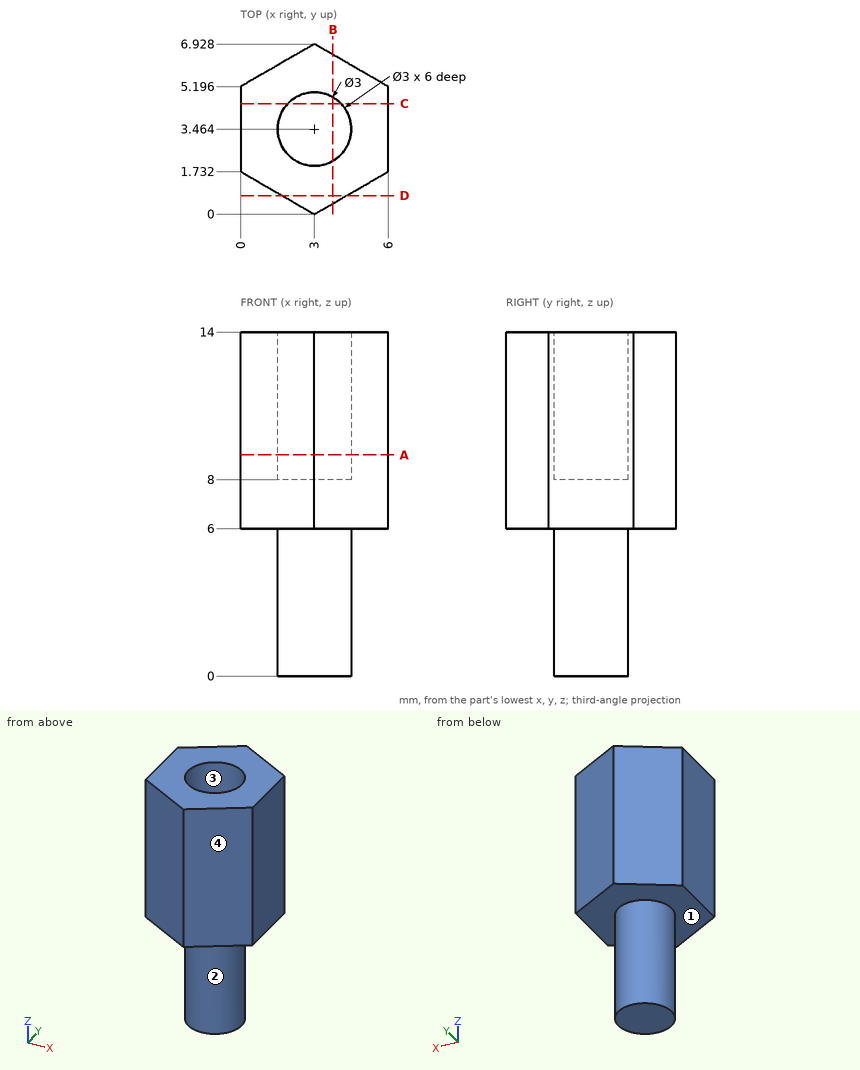
Geometry check sheet. Reference: drawing and pictorial views, mm from the part's lowest x, y, z. Coordinates: 2 decimals unless noted, no trailing zeros. Order: outer loops, then holes, each group sorted by start corner. A loop starts at its lowest first (then second) coordinate and runs counter-clockwise, first axis right, second up.
Item 1: Depth check by flat-ended pin: pin 1 (1.5 mm diameter, centred on x = 2.5, y = 3.5, fed in from +Z); pin 2 (1 mm diameter, centred on x = 1.5, y = 5.5, fed in from -Z). Enter the tip coordinate at first touch or a pass-through.
Item 2: Section check A-A (z = 9). Enter the section's corners in (x, y), plus the area to 3 significant figures.
Item 3: Mould release check, pull along X, two halves, no side actions. Record for the marked faces 1, 2, 3 and 4: released by +X, released by -X, zero draft, split by the parting line, or undercut.
Item 4: Section check B-B (x = 3.75). Enter the section's corners in (y, z) (1 decimal), plus the area to 3 significant figures.
Item 5: Section check D-D (y = 0.75). Enter the section's corners in (x, z).
Item 6: Section check C-C (y = 4.5). Enter the section's corners in (x, z) (1 decimal), plus the area to 3 significant figures.
Item 7: Scan lines: line 1 along Z through (x, y) = (0.5, 5); line 2 along X through (y, z) = (4.5, 8.5) (1 decimal); line 3 along Y through (x, z) = (3, 3.5). Record each from-to range of solid material in increasing order.
Check sheet entries:
1. pin 1: stops at z = 8
1. pin 2: stops at z = 6
2. outline: (0, 1.73) - (3, 0) - (6, 1.73) - (6, 5.2) - (3, 6.93) - (0, 5.2) - close; hole circle Ø3 at (3, 3.46)
2. area: 24.1 mm2
3. face 1: zero draft
3. face 2: split by the parting line
3. face 3: undercut
3. face 4: released by +X
4. outline: (0.4, 6) - (2.2, 6) - (2.2, 0) - (4.8, 0) - (4.8, 6) - (6.5, 6) - (6.5, 14) - (4.8, 14) - (4.8, 8) - (2.2, 8) - (2.2, 14) - (0.4, 14) - close
4. area: 48.5 mm2
5. outline: (1.7, 6) - (4.3, 6) - (4.3, 14) - (1.7, 14) - close
6. outline: (0, 6) - (1.9, 6) - (1.9, 0) - (4.1, 0) - (4.1, 6) - (6, 6) - (6, 14) - (4.1, 14) - (4.1, 8) - (1.9, 8) - (1.9, 14) - (0, 14) - close
6. area: 48.0 mm2
7. line 1: z = 6 to 14
7. line 2: x = 0 to 1.9, 4.1 to 6
7. line 3: y = 1.96 to 4.96
